```python
from build123d import *

# Parameters (mm, degrees)
CROQUIS1_R              = 4
SALIENTE_EXTRUIR1_DEPTH = 3
CROQUIS2_R              = 4
SALIENTE_EXTRUIR2_DEPTH = 3
CROQUIS3_W              = 31
CROQUIS3_H              = 49.380731332
SALIENTE_EXTRUIR3_DEPTH = 3
CROQUIS5_R              = 4
CORTAR_EXTRUIR1_DEPTH   = 3


with BuildPart() as part:
    # Croquis1 → Saliente-Extruir1 (new body)
    with BuildSketch(Plane(origin=(0, 0, 0), x_dir=(0, 0, -1), z_dir=(1, 0, 0))):
        with BuildLine():
            Line((-9.335804265, -3.583679495), (-24.690365666, 36.416320505))
            Line((-24.690365666, 36.416320505), (24.690365666, 36.416320505))
            Line((24.690365666, 36.416320505), (9.335804265, -3.583679495))
            ThreePointArc((9.335804265, -3.583679495), (0, -10), (-9.335804265, -3.583679495))
        make_face()
        Circle(CROQUIS1_R, mode=Mode.SUBTRACT)
    extrude(amount=SALIENTE_EXTRUIR1_DEPTH)



with BuildPart() as body_2:
    # Croquis2 → Saliente-Extruir2 (new body)
    with BuildSketch(Plane.ZY.offset(25)):
        with BuildLine():
            Line((9.335804265, -3.583679495), (24.690365666, 36.416320505))
            Line((24.690365666, 36.416320505), (-24.690365666, 36.416320505))
            Line((-24.690365666, 36.416320505), (-9.335804265, -3.583679495))
            ThreePointArc((-9.335804265, -3.583679495), (0, -10), (9.335804265, -3.583679495))
        make_face()
        Circle(CROQUIS2_R, mode=Mode.SUBTRACT)
    extrude(amount=SALIENTE_EXTRUIR2_DEPTH)


with BuildPart() as part_1:
    add(part.part)

    add(body_2.part)  # Saliente-Extruir3 merges body 2
    # Croquis3 → Saliente-Extruir3 (add)
    with BuildSketch(Plane(origin=(0, 36.416320505, 0), x_dir=(1, 0, 0), z_dir=(0, 1, 0))):
        with Locations((-12.5, 0)):
            Rectangle(CROQUIS3_W, CROQUIS3_H)
    extrude(amount=SALIENTE_EXTRUIR3_DEPTH)

    # Croquis5 → Cortar-Extruir1 (cut)
    with BuildSketch(Plane(origin=(0, 39.416320505, 0), x_dir=(1, 0, 0), z_dir=(0, 1, 0))):
        with Locations((-12.5, 0)):
            Circle(CROQUIS5_R)
    extrude(amount=-CORTAR_EXTRUIR1_DEPTH, mode=Mode.SUBTRACT)


solid = part_1.part
```
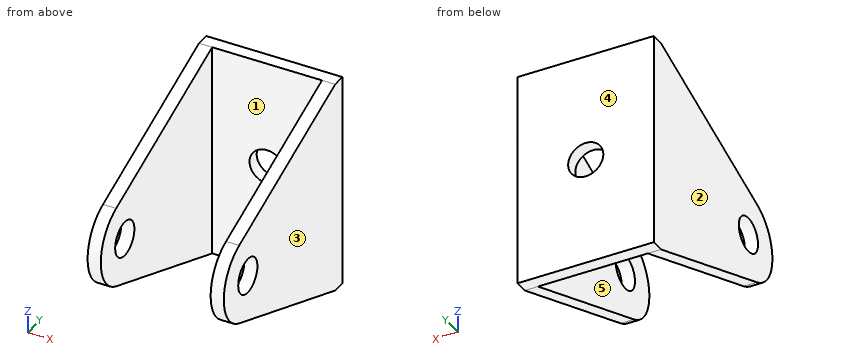
CAD build for the part. Positions are in the model's coordinates, mm. Face numbers are marked on the shaded views. A direction names the side the tool comes from. Coordinates: 2 decimals unless noted, no trailing zeros. Order: outer loops, then holes, each group sorted by start corner. A loop starts at its lowest first (then second) coordinate and runs counter-clockwise, first axis right, second up. Notation, with made-up numbers: (-38.5, -2) -> (-21.5, -2) arc R36 ccw to (-21.5, 32) -> close; hole circle Ø9 at (-21.75, 17). An arc over 180 degrees is marked (long way). Use one line per item in the form item = value. Start each with the question number.
1) Tool access for the marked faces 4 and 5: list every direction of +Z, -Z, +X, -X, +Y, -Y with a clear straight run to the whole face (end or side of a thin tool).
2) Band-saw the part on D-D on x = 1.5. Give the cut face in (y, z), then the cut area to 3 significant figures.
3) Band-saw the part on A-A on z = 0. Give the cut face in (x, y).
4) Pull direction X, two halves, no side cores. Call the marked faces 1, 2 and 3: +X half, -X half, draft (parallel to the pull), parting line (faces both ways), or undercut.
5) Drill centre lines: L1, parallel to X at y = 27.5, z = -19; L2, parallel to X at y = 37.5, z = 0; L3, parallel to Y at x = -19, z = 11.5. Where is each one in solid material? Low to high. Write a range as [from, to].
6) Band-saw the part on B-B on x = -12.5. Give the cut face in (y, z).
7) Drop a flat-ended pin along its axis: pin 1 (5 mm diameter, centred on x = -9, z = -13, fed in from -Y). Give the stop position or say it passes through.
8) Band-saw the part on C-C on y = -2.5. Give the cut face in (x, z), then the cut area to 3 significant figures.
Entries:
q1.face_4 = +Z, -Z, +X, -X, +Y
q1.face_5 = +Z, -Z, -Y
q2.outline = (-3.58, -9.34) -> (36.42, -24.69) -> (39.42, -24.69) -> (39.42, 24.69) -> (36.42, 24.69) -> (-3.58, 9.34) arc R10 ccw to start; hole circle Ø8 at (0, 0)
q2.area = 1,550 mm2
q3.outline = (-28, -10) -> (-25, -10) -> (-25, -4) -> (-28, -4) -> close; (-28, 4) -> (-25, 4) -> (-25, 36.42) -> (-16.5, 36.42) -> (-16.5, 39.42) -> (-28, 39.42) -> close; (-8.5, 36.42) -> (0, 36.42) -> (0, 4) -> (3, 4) -> (3, 39.42) -> (-8.5, 39.42) -> close; (0, -10) -> (3, -10) -> (3, -4) -> (0, -4) -> close
q4.face_1 = undercut
q4.face_2 = -X half
q4.face_3 = +X half
q5.L1 = [-28, -25], [0, 3]
q5.L2 = [-28, -16.5], [-8.5, 3]
q5.L3 = [36.42, 39.42]
q6.outline = (36.42, -24.69) -> (39.42, -24.69) -> (39.42, -4) -> (36.42, -4) -> close; (36.42, 4) -> (39.42, 4) -> (39.42, 24.69) -> (36.42, 24.69) -> close
q7.pin_1 = 36.42
q8.outline = (-28, -9.75) -> (-25, -9.75) -> (-25, -3.12) -> (-28, -3.12) -> close; (-28, 3.12) -> (-25, 3.12) -> (-25, 9.75) -> (-28, 9.75) -> close; (0, -9.75) -> (3, -9.75) -> (3, -3.12) -> (0, -3.12) -> close; (0, 3.12) -> (3, 3.12) -> (3, 9.75) -> (0, 9.75) -> close
q8.area = 79.6 mm2
